Could you check a few things on this model? Use its own coordinates, in mm. A direction names the side the tool comes from. Give positions to 0.01 mm unless a question says otherwise; leave off trailing zeros. Order: outer loops, then holes, each group sorted by start corner. A loop starts at its lowest first (then second) coordinate and runs counter-clockwise, first axis right, second up. Notation, with made-up numbers: M -21,18.5 L 19,18.5 A18 cw 19,34.5 Z; hole C 75,69 d7. An arc over 180 degrees is marked long. Return JSON: item names as keys, results as strings. Group by question number.
```python
from build123d import *

# Parameters (mm, degrees)
F0_W     = 3.81
F0_H     = 3.81
F1_DEPTH = 11.43
F2_W     = 3.5260741734
F2_H     = 220.98
F3_DEPTH = 25.4
F4_W     = 3.5260741734
F4_H     = 3.81
F5_DEPTH = 3.81
F6_W     = 3.81
F6_H     = 3.81
F7_DEPTH = 25.4


with BuildPart() as f1:
    # F0 (on Right) → F1 (new body)
    with BuildSketch(Plane.YZ):
        with Locations((-41.9773963976, -0.0329993901)):
            Rectangle(F0_W, F0_H)
        with Locations((-38.1673963976, -0.0329993901)):
            Rectangle(F0_W, F0_H)
        Polygon((-40.0723963976, -1.9379993901), (-43.8823963976, -1.9379993901), (-43.8823963976, -212.0072897974), (-40.0723963976, -197.7881762206), align=None)
        with Locations((-34.3573963976, -0.0329993901)):
            Rectangle(F0_W, F0_H)
        Polygon((-40.0723963976, -197.7881762206), (-43.8823963976, -212.0072897974), (-43.8823963976, -226.7279993901), (-40.0723963976, -212.5088858132), align=None)
        Polygon((-32.4523963976, -1.9379993901), (-36.2623963976, -1.9379993901), (-36.2623963976, -183.5690626437), (-32.4523963976, -169.3499490669), align=None)
        Polygon((-36.2623963976, -183.5690626437), (-40.0723963976, -197.7881762206), (-40.0723963976, -212.5088858132), (-36.2623963976, -198.2897722364), align=None)
        Polygon((-32.4523963976, -169.3499490669), (-36.2623963976, -183.5690626437), (-36.2623963976, -198.2897722364), (-32.4523963976, -184.0706586596), align=None)
    extrude(amount=F1_DEPTH)

    # F2 (on face) → F3 (cut)
    with BuildSketch(Plane.XZ.offset(43.8823963976)):
        with Locations((5.5730370867, -112.4279993901)):
            Rectangle(F2_W, F2_H)
    extrude(amount=-F3_DEPTH, mode=Mode.SUBTRACT)

    # F4 (on face) → F5 (join)
    with BuildSketch(Plane(origin=(0, -32.4523963976, 0), x_dir=(-1, 0, 0), z_dir=(0, 1, 0))):
        with Locations((-5.5730370867, -182.1656586596)):
            Rectangle(F4_W, F4_H)
    extrude(amount=-F5_DEPTH)

    # F6 (on face) → F7 (cut)
    with BuildSketch(Plane.XY.offset(1.8720006099)):
        with Locations((5.715, -38.1673963976)):
            Rectangle(F6_W, F6_H)
    extrude(amount=-F7_DEPTH, mode=Mode.SUBTRACT)


solid = f1.part
```
1. Imagine slicing it at B-B, the plane x = 9.5. Please give me the cut outline in (y, z).
2. I need wall thicknesses on L1, parallel to Y at x = 9.75, z = -95; L2, parallel to X at y = -43, z = -38; L3, parallel to Y at x = 0.5, z = -194. Which ranges of each line are inside material? Lowest first, please. Write a range as from..to.
3. Imagine slicing it at A-A, the plane z = -55. Please give me the cut outline in (x, y).
4. For pin 1 (1.8 mm diameter, centred on x = 5, y = -34, fed in from -Z); pin 2 (5.5 mm diameter, centred on x = 5.5, z = -78, fed in from -Y); pin 3 (1.1 mm diameter, centred on x = 6, y = -41, fed in from -Z), each with a flat end and sliding along its axis, tell me the tip position at first contact or that it passes through.
5. Imagine slicing it at C-C, the plane z = -201. Please give me the cut outline in (x, y).
6. If we mould it in two halves opening along X, with no side actions, what happens to faces 6 (the flat face through (0, -41, -111)), 7 (the flat face through (6, -42, -1.938)), 8 (the flat face through (3, -43.882, -111))? For each: pulls with the +X half, pulls with the -X half, needs draft (parallel to the pull), parting line crosses it, or undercut.
7. Which directions (+Z, -Z, +X, -X, +Y, -Y) give clear straight access to the entire face, cutting with the end or side of a thin tool? Please do faces 1 (the flat face through (7.62, -38, 0)), 2 (the flat face through (7.336, -34, -92)), 3 (the flat face through (3.81, -38, 0)), 4 (the flat face through (11.43, -41, -111)), 5 (the flat face through (2, -40.072, -101)).
Values:
{
 "1": {"outline": "M -43.88,-226.73 L -32.45,-184.07 L -32.45,1.87 L -43.88,1.87 Z; hole M -40.07,-197.79 L -36.26,-183.57 L -36.26,-1.94 L -40.07,-1.94 Z"},
 "2": {"L1": "y = -43.88..-40.07, -36.26..-32.45", "L2": "x = 0..3.81, 7.34..11.43", "L3": "y = -43.88..-40.07, -39.06..-35.11"},
 "3": {"outline": "M 0,-43.88 L 3.81,-43.88 L 3.81,-40.07 L 0,-40.07 Z; M 0,-36.26 L 3.81,-36.26 L 3.81,-32.45 L 0,-32.45 Z; M 7.34,-43.88 L 11.43,-43.88 L 11.43,-40.07 L 7.34,-40.07 Z; M 7.34,-36.26 L 11.43,-36.26 L 11.43,-32.45 L 7.34,-32.45 Z"},
 "4": {"pin 1": "stops at z = -184.07", "pin 2": "stops at y = -43.88", "pin 3": "stops at z = -1.94"},
 "5": {"outline": "M 0,-43.88 L 3.81,-43.88 L 3.81,-36.99 L 0,-36.99 Z; M 7.34,-43.88 L 11.43,-43.88 L 11.43,-36.99 L 7.34,-36.99 Z"},
 "6": {"face 6": "pulls with the -X half", "face 7": "undercut", "face 8": "needs draft"},
 "7": {"face 1": "+Z", "face 2": "+Y, -Y", "face 3": "+Z, -Z", "face 4": "+Z, -Z, +X, +Y, -Y", "face 5": "+X, -X"}
}
